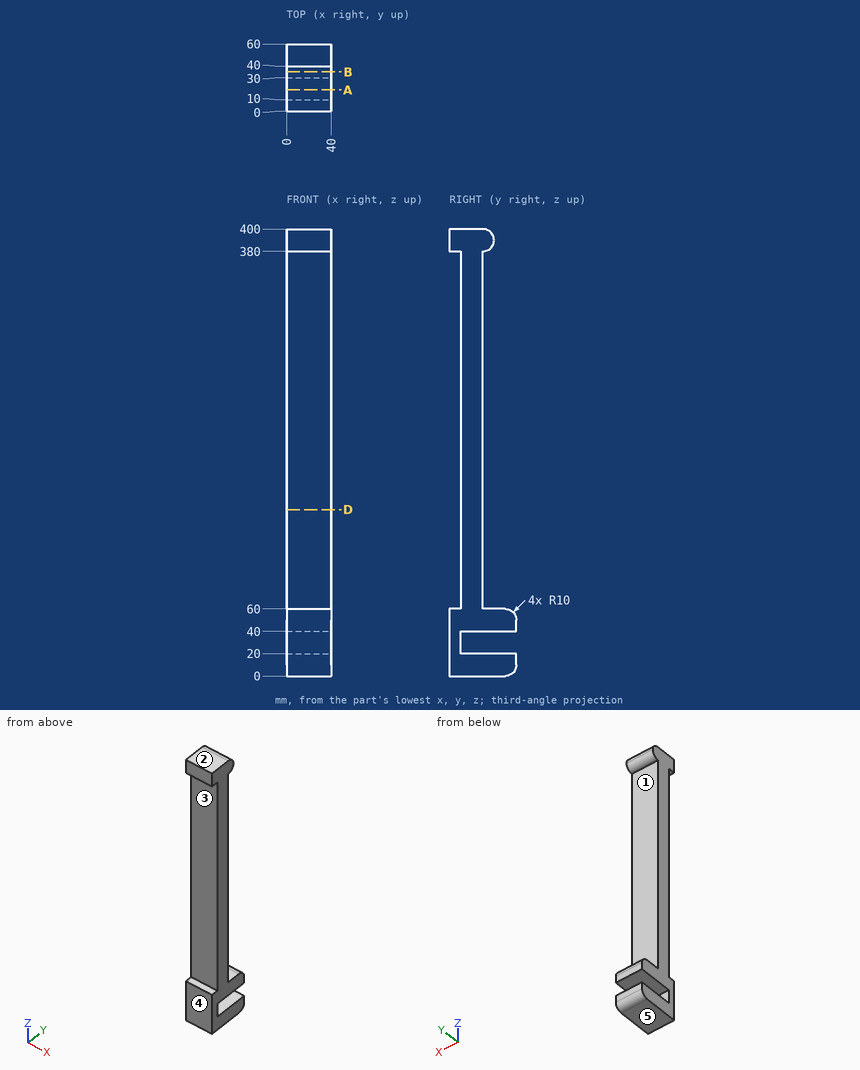
Geometry check sheet. Reference: drawing and pictorial views, mm from the part's lowest x, y, z. A direction names the side the tool comes from. Round coordinates to 2 decimals unless told otherwise and drop trailing zeros. Loops run counter-clockwise (first coordinate to the right, second up) from the corner with the lowest first, then second, coordinate; pieces in that order, holes last. Notation, with made-up numbers: M -22,-8.5 L 19,-8.5 A17 ccw 19,22.5 Z; hole C 9.25,-20.75 d6. An arc over 180 degrees is marked long. One line per item, written item: value.
(1) Sectioned sample at B-B, the plane y = 35. Record the cut outline in (x, z), then the cut area to 3 significant figures.
Computed values:
outline: M 0,0 L 40,0 L 40,20 L 0,20 Z; M 0,40 L 40,40 L 40,60 L 0,60 Z; M 0,381.34 L 40,381.34 L 40,398.66 L 0,398.66 Z
area: 2,290 mm^2
(2) Thickness scan on line 1 (Z direction, x = 14.5, y = 27); line 2 (Z direction, x = 30, y = 43.5); line 3 (Y direction, x = 9, z = 94.5). Record the ranges inside material, lowest first.
Computed values:
line 1: z = 0 to 20, 40 to 400
line 2: z = 0 to 20, 40 to 60
line 3: y = 10 to 30
(3) Sectioned sample at A-A, the plane y = 19. Record the cut outline in (x, z), then the cut area to 3 significant figures.
Computed values:
outline: M 0,0 L 40,0 L 40,20 L 0,20 Z; M 0,40 L 40,40 L 40,400 L 0,400 Z
area: 15,200 mm^2
(4) Access from +Z, -Z, +X, -X, +Y, -Y to the whole of each face (thin tool, end or side, straight path). Record for the marked faces 1 and 2.
Computed values:
face 1: +X, -X, +Y
face 2: +Z, +X, -X, +Y, -Y
(5) Sectioned sample at D-D, the plane z = 149. Record the cut outline in (x, y).
Computed values:
outline: M 0,10 L 40,10 L 40,30 L 0,30 Z
(6) Release check for a two-part mould opening along Z. For the marked faces 3, 4 and 5 record: +Z half, -Z half, draft (parallel to the pull), parting line (faces both ways), or undercut.
Computed values:
face 3: undercut
face 4: draft
face 5: -Z half
(7) Depth check by flat-ended pin: pin 1 Ø12 at (x, z) = (13, 201.5) entering from -Y; pin 2 Ø10 at (x, z) = (27.5, 30.5) entering from +Y; pin 3 Ø2 at (x, z) = (6, 307) entering from +Y. Enter the tip coordinate at first touch or a pass-through.
Computed values:
pin 1: stops at y = 10
pin 2: stops at y = 10
pin 3: stops at y = 30
